Build history of the part. All positions in model axes, mm. Face numbers are marked on the shaded views. A direction names the side the tool comes from. Coordinates: 2 decimals unless noted, no trailing zeros. Loops run counter-clockwise (first coordinate to the right, second up) from the corner with the lowest first, then second, coordinate; pieces in that order, holes last. Notation, with made-up numbers: (74, 4) -> (95, 4) arc R24 cw to (95, 16) -> close; hole circle Ø8 at (7, 22). An arc over 180 degrees is marked (long way). One line per item, written item: value. Start each with the question number.
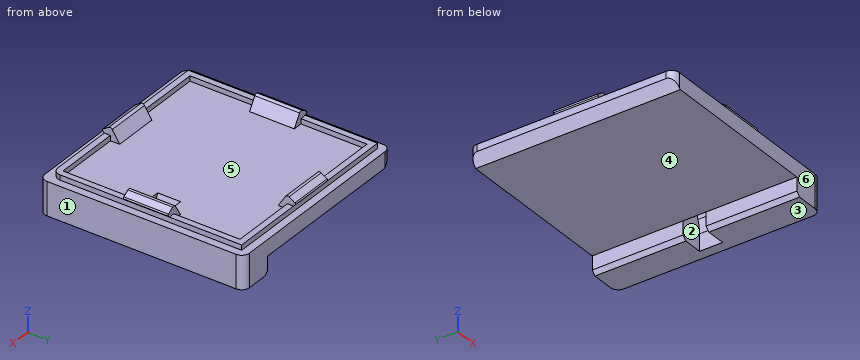
```python
from build123d import *

# Parameters (mm, degrees)
SKETCH_W           = 80
SKETCH_H           = 80
PAD_DEPTH          = 13
PAD001_DEPTH       = 8.75
POLARPATTERN_COUNT = 4
SKETCH006_W        = 67
SKETCH006_H        = 6.8
POCKET_DEPTH       = 40.001
POCKET_DEPTH_BACK  = 40.001
SKETCH008_W        = 9
SKETCH008_H        = 9
CHAMFER_SIZE       = 3.5
FILLET_R           = 3
CHAMFER002_SIZE    = 1.5
SKETCH014_W        = 74
SKETCH014_H        = 74
SKETCH014_W_2      = 69.2
SKETCH014_H_2      = 69.2
PAD005_DEPTH       = 2
FILLET003_R        = 3


with BuildPart() as part:
    # Sketch → Pad (new body)
    with BuildSketch(Plane.XY):
        Rectangle(SKETCH_W, SKETCH_H)
    extrude(amount=-PAD_DEPTH)

    # Sketch001 → Pad001 (join, symmetric)
    with BuildSketch(Plane.YZ):
        with BuildLine():
            Line((31, 0), (33.85683, 4.513208))
            ThreePointArc((35.236626, 4.82331), (34.482504, 4.954025), (33.85683, 4.513208))
            Line((35.236626, 4.82331), (37.517423, 3.379581))
            ThreePointArc((37.603553, 2.603553), (37.746949, 3.012262), (37.517423, 3.379581))
            Line((37.603553, 2.603553), (37, 2))
            Line((37, 2), (37, 0))
            Line((37, 0), (31, 0))
        make_face()
    pad001 = extrude(amount=PAD001_DEPTH, both=True)

    # PolarPattern: Pad001 ×4 about axis
    polarpattern_axis = Axis((0, 0, 0), (0, 0, 1))
    for i in range(1, POLARPATTERN_COUNT):
        add(pad001.rotate(polarpattern_axis, i * 360 / POLARPATTERN_COUNT))

    # Sketch006 → Pocket (cut, two sides)
    with BuildSketch(Plane.XZ) as pocket_sk:
        with Locations((-6.5, -9.6)):
            Rectangle(SKETCH006_W, SKETCH006_H)
    extrude(amount=-POCKET_DEPTH, mode=Mode.SUBTRACT)
    extrude(pocket_sk.sketch, amount=POCKET_DEPTH_BACK, mode=Mode.SUBTRACT)

    # SubtractivePipe: sweep along a path in Sketch009
    with BuildLine(Plane.XZ) as subtractivepipe_path:
        Line((31.5, -13), (31.5, -6.420201))
        ThreePointArc((31.5, -6.420201), (31.348078, -4.68372), (30.896926, -3))
        Line((30.896926, -3), (26.165313, 10))
    # Sketch008 (on Face4 of Pocket) → SubtractivePipe (sweep, cut)
    with BuildSketch(Plane(origin=(0, 0, -13), x_dir=(1, 0, 0), z_dir=(0, 0, -1))):
        with Locations((31.5, 0)):
            Rectangle(SKETCH008_W, SKETCH008_H)
    sweep(path=subtractivepipe_path.line, mode=Mode.SUBTRACT)

    # Chamfer
    chamfer_edges = [part.edges().sort_by_distance(p)[0] for p in [
        (-40, 0, -6.2),
    ]]
    chamfer(chamfer_edges, length=CHAMFER_SIZE)

    # Fillet
    fillet_edges = [part.edges().sort_by_distance(p)[0] for p in [
        (40, -40, -6.5),
        (40, 40, -6.5),
        (-40, 40, -1.35),
        (-40, -40, -1.35),
    ]]
    fillet(fillet_edges, radius=FILLET_R)

    # Chamfer002
    chamfer002_edges = [part.edges().sort_by_distance(p)[0] for p in [
        (27, 22.25, -13),
        (27, -22.25, -13),
    ]]
    chamfer(chamfer002_edges, length=CHAMFER002_SIZE)

    # Sketch014 → Pad005 (join)
    with BuildSketch(Plane.XY):
        Rectangle(SKETCH014_W, SKETCH014_H)
        Rectangle(SKETCH014_W_2, SKETCH014_H_2, mode=Mode.SUBTRACT)
    extrude(amount=PAD005_DEPTH)

    # Fillet003
    fillet003_edges = [part.edges().sort_by_distance(p)[0] for p in [
        (-35.236626, 0, 4.82331),
        (37, -37, 1),
        (0, -35.236626, 4.82331),
        (0, 35.236626, 4.82331),
    ]]
    fillet(fillet003_edges, radius=FILLET003_R)


solid = part.part
```
Item 1: Drop flat-ended pins along their axis: pin 1 Ø2.5 at (y, z) = (34, 2.5) entering from -X; pin 2 Ø22.5 at (x, y) = (-19.5, 25) entering from +Z; pin 3 Ø3 at (x, y) = (-24.5, 14.5) entering from -Z. Give the stop position or say it passes through.
Item 2: Band-saw the part on D-D, the plane y = 15. List the corners of the cut face in (x, z).
Item 3: Tool access for the marked faces 4, 5 and 6: list every direction of +Z, -Z, +X, -X, +Y, -Y with a clear straight run to the whole face (end or side of a thin tool).
Item 4: Probe probe 1 along X at (y, z) = (27, 0.5); probe 2 along Z at (x, y) = (-19.5, 28). List the from-to ranges inside material, lowest first.
Item 5: Band-saw the part on B-B, the plane x = -18. List the corners of the cut face in (y, z), and give its area (3 significant figures).
Item 6: Band-saw the part on A-A, the plane y = 1. List the corners of the cut face in (x, z), and give its area (3 significant figures).
Item 7: Band-saw the part on C-C, the plane z = -7.5. List the corners of the cut face in (x, y).
Item 8: Two-plate mould, pull along X, no slides. Class the marked faces 1, 2 and 3: +X half, -X half, draft (parallel to the pull), parting line (faces both ways), or undercut.
Worked out:
1. pin 1: stops at x = -37
1. pin 2: stops at z = 2
1. pin 3: stops at z = -6.2
2. outline: (-40, -2.7) -> (-36.5, -6.2) -> (27, -6.2) -> (27, -11.5) -> (28.5, -13) -> (40, -13) -> (40, 0) -> (37, 0) -> (37, 2) -> (34.6, 2) -> (34.6, 0) -> (-34.6, 0) -> (-34.6, 2) -> (-37, 2) -> (-37, 0) -> (-40, 0) -> close
3. face 4: -Z, -X, +Y, -Y
3. face 5: +Z
3. face 6: +Z, -Z, +X, -X, -Y
4. probe 1: x = -37 to -34.6, 34.6 to 37
4. probe 2: z = -6.2 to 0
5. outline: (-40, -6.2) -> (40, -6.2) -> (40, 0) -> (37, 0) -> (37, 2) -> (34.6, 2) -> (34.6, 0) -> (-34.6, 0) -> (-34.6, 2) -> (-37, 2) -> (-37, 0) -> (-40, 0) -> close
5. area: 506 mm²
6. outline: (-40, -2.7) -> (-36.5, -6.2) -> (27, -6.2) arc R5.5 ccw to (26.67, -4.54) -> (25.02, 0) -> (-31, 0) -> (-33.86, 4.51) arc R1 ccw to (-35.24, 4.82) -> (-37.52, 3.38) arc R0.5 ccw to (-37.6, 2.6) -> (-37, 2) -> (-37, 0) -> (-40, 0) -> close; (33.28, 3.6) -> (35.13, -1.46) arc R14.5 cw to (36, -6.42) -> (36, -13) -> (40, -13) -> (40, 0) -> (37, 0) -> (37, 2) -> (37.6, 2.6) arc R0.5 ccw to (37.52, 3.38) -> (35.24, 4.82) arc R1 ccw to (33.86, 4.51) -> close
6. area: 495 mm²
7. outline: (27, -40) -> (37, -40) arc R3 ccw to (40, -37) -> (40, 37) arc R3 ccw to (37, 40) -> (27, 40) -> (27, 4.5) -> (36, 4.5) -> (36, -4.5) -> (27, -4.5) -> close
8. face 1: +X half
8. face 2: undercut
8. face 3: draft
